```python
from build123d import *

# Parameters (mm, degrees)
F0_R     = 9.92251
F0_W     = 76.2
F0_H     = 7.9375
F1_DEPTH = 88.9
F2_W     = 73.025
F2_H     = 65.0875
F3_DEPTH = 63.5
F4_R     = 10.3251
F5_DEPTH = 25.4


with BuildPart() as f1:
    # F0 (on Front) → F1 (new body)
    with BuildSketch(Plane.XZ):
        with BuildLine():
            ThreePointArc((57.15, 44.45), (28.575, 73.025), (0, 44.45))
            Line((0, 44.45), (0, 0))
            Line((0, 0), (57.15, 0))
            Line((57.15, 0), (57.15, 7.9375))
            Line((57.15, 7.9375), (57.15, 44.45))
        make_face()
        with Locations((28.575, 44.45)):
            Circle(F0_R, mode=Mode.SUBTRACT)
        with Locations((95.25, 3.96875)):
            Rectangle(F0_W, F0_H)
    extrude(amount=F1_DEPTH)

    # F2 (on Right) → F3 (cut)
    with BuildSketch(Plane.YZ):
        with Locations((-44.45, 40.48125)):
            Rectangle(F2_W, F2_H)
    extrude(amount=F3_DEPTH, mode=Mode.SUBTRACT)

    # F4 (on Top) → F5 (cut)
    with BuildSketch(Plane.XY):
        with Locations((73.025, -44.45)):
            Circle(F4_R)
        with Locations((111.125, -44.45)):
            Circle(F4_R)
        with BuildLine():
            Line((57.15, -88.9), (133.35, -88.9))
            Line((133.35, -88.9), (133.35, -44.45))
            ThreePointArc((133.35, -44.45), (126.840448, -60.165448), (111.125, -66.675))
            Line((111.125, -66.675), (63.5, -66.675))
            ThreePointArc((63.5, -66.675), (59.009872, -68.534872), (57.15, -73.025))
            Line((57.15, -73.025), (57.15, -88.9))
        make_face()
        with BuildLine():
            ThreePointArc((111.125, -22.225), (126.840448, -28.734552), (133.35, -44.45))
            Line((133.35, -44.45), (133.35, 0))
            Line((133.35, 0), (57.15, 0))
            Line((57.15, 0), (57.15, -15.875))
            ThreePointArc((57.15, -15.875), (59.009872, -20.365128), (63.5, -22.225))
            Line((63.5, -22.225), (111.125, -22.225))
        make_face()
    extrude(amount=F5_DEPTH, mode=Mode.SUBTRACT)


solid = f1.part
```
Here's how the part is built. I have some questions about the finished solid (model axes, mm). A direction names the side the tool comes from. Coordinates: 2 decimals unless noted, no trailing zeros. Write each loop counter-clockwise with the first axis right and the second up, starting at its lowest first coordinate (ties: lowest second). Pieces come first, ordered by that corner, then holes. Notation, with made-up numbers: (-4, 16.25) -> (6, 16.25) arc R27 ccw to (6, 42.25) -> close; hole circle Ø2 at (-30.75, 64). An arc over 180 degrees is marked (long way). Use a Markdown table: item, result. Add a question column.
(1) I'm going to push flat-ended pins straight in: P1, Ø8, axis at y = -4, z = 30, coming from the +X side; P2, Ø2.5, axis at x = 75.5, z = 5.5, coming from the +Y side (3 decimals); P3, Ø6.5, axis at x = 85, z = 4, coming from the -Y side (3 decimals). Where does each tip first touch, or does it pass through?
(2) If we section it at A-A, the plane z = 12: Write out the boundary of the cut face in (x, y), and give its area (3 significant figures).
(3) For faces 1 (the flat face through (51, -44, 7.938)), 2 (the flat face through (88, -66.675, 4)), 3 (the cylindrical face through (29.2, -3.91, 73.02)), which set-ups out of +Z, -Z, +X, -X, +Y, -Y let a thin tool reach every point of the face, with its end or its side?
(4) Please list where these lines run through material, in increasing order: line 1 (Y direction, x = 32, z = 65); line 2 (X direction, y = -2, z = 44); line 3 (Z direction, x = 61, y = -33.5).
(5) If we section it at D-D, the plane x = 17: Write out the boundary of the cut face in (y, z).
(6) If we section it at B-B, the plane x = 67: Write out the boundary of the cut face in (y, z) (1 decimal), and give its area (3 significant figures).
(7) If we section it at C-C, the plane z = 43: Write out the boundary of the cut face in (x, y), and give its area (3 significant figures).
(8) We'd pull the mould along Y, two halves only. Please class faces 4 (the cylindrical face through (120.973, -41.349, 3.913)), 5 (the flat face through (87, -22.225, 4)), 6 (the flat face through (0, -43.8, 7.7)): +Y half, -Y half, draft (parallel to the pull), parting line (faces both ways), or undercut.
Outcome:
| question | item | result |
|---|---|---|
| 1 | P1 | stops at x = 57.15 |
| 1 | P2 | stops at y = -22.225 |
| 1 | P3 | stops at y = -66.675 |
| 2 | outline | (0, -88.9) -> (57.15, -88.9) -> (57.15, -80.96) -> (0, -80.96) -> close; (0, -7.94) -> (57.15, -7.94) -> (57.15, 0) -> (0, 0) -> close |
| 2 | area | 907 mm^2 |
| 3 | face 1 | +Z, +X, -X |
| 3 | face 2 | +Z, -Z, +X, -Y |
| 3 | face 3 | +Z, +Y, -Y |
| 4 | line 1 | y = -88.9 to -80.96, -7.94 to 0 |
| 4 | line 2 | x = 0 to 18.66, 38.49 to 57.15 |
| 4 | line 3 | z = 0 to 7.94 |
| 5 | outline | (-88.9, 0) -> (0, 0) -> (0, 70.58) -> (-7.94, 70.58) -> (-7.94, 7.94) -> (-80.96, 7.94) -> (-80.96, 70.58) -> (-88.9, 70.58) -> close |
| 6 | outline | (-66.7, 0) -> (-52.8, 0) -> (-52.8, 7.9) -> (-66.7, 7.9) -> close; (-36.1, 0) -> (-22.2, 0) -> (-22.2, 7.9) -> (-36.1, 7.9) -> close |
| 6 | area | 220 mm^2 |
| 7 | outline | (0, -88.9) -> (18.76, -88.9) -> (18.76, -80.96) -> (0, -80.96) -> close; (0, -7.94) -> (18.76, -7.94) -> (18.76, 0) -> (0, 0) -> close; (38.39, -88.9) -> (57.15, -88.9) -> (57.15, -80.96) -> (38.39, -80.96) -> close; (38.39, -7.94) -> (57.15, -7.94) -> (57.15, 0) -> (38.39, 0) -> close |
| 7 | area | 596 mm^2 |
| 8 | face 4 | undercut |
| 8 | face 5 | +Y half |
| 8 | face 6 | draft |
